Design review of the part built by this model. Coordinates are the model's own, in mm. Round coordinates to 2 decimals unless told otherwise and drop trailing zeros. Loops run counter-clockwise (first coordinate to the right, second up) from the corner with the lowest first, then second, coordinate; pieces in that order, holes last. Notation, with made-up numbers: M 83,-8 L 89,-8 A18 cw 89,19 Z; hole C 59.5,45 d1. An arc over 180 degrees is marked long. One line per item, written item: value. Start each with the question number.
Item 1: We need section C-C (y = 8). Write out the cut boundary in (x, z), then the cut area to 3 significant figures.
Item 2: We need section B-B (x = 0). Write out the cut boundary in (y, z), then the cut area to 3 significant figures.
Item 3: Clearance check with a flat-ended pin moving along its axis: pin 1 (2 mm diameter, centred on x = -4, y = -1, fed in from -Z). State where the tip first meets the part, or that it passes through.
Item 4: For line 1 along Y through (x, z) = (0.25, 1.25); line 2 along Y through (x, z) = (-8.75, 0.5); line 3 along Y through (x, z) = (-6, 0.9), list the stretches that pass through material, from the lowest coordinate up.
Item 5: We need section D-D (x = -8). Write out the cut boundary in (y, z).
Item 6: We need section A-A (y = 0). Write out the cut boundary in (x, z).
Autodesk Inventor part; units mm, degrees
ref_plane "YZ Plane" through (0, 0, 0) normal (1, 0, 0) x (0, 1, 0)
ref_plane "XZ Plane" through (0, 0, 0) normal (0, 1, 0) x (-1, 0, 0)
ref_plane "XY Plane" through (0, 0, 0) normal (0, 0, 1) x (1, 0, 0)
sketch "Sketch1" plane through (0, 0, 0) normal (0, 0, 1) x (1, 0, 0)
  circle A0 centre (0, 0) radius 40
  circle A1 centre (0, -8) radius 1.5
  circle A2 centre (8, 0) radius 1.5
  circle A3 centre (0, 8) radius 1.5
  circle A4 centre (-8, 0) radius 1.5
  circle A5 centre (0, -34) radius 1.5
  circle A6 centre (-3.0155, -32.086) radius 0.5
  circle A7 centre (2.9845, -36.086) radius 0.5
  line L0 (-15, -37.081) -> (-15, 37.081)
  line L1 (15, -37.081) -> (15, 37.081)
  dimension "d0" = 80
  dimension "d1" = 8
  dimension "d2" = 3
  dimension "d5" = 360
  dimension "d9" = 3
  dimension "d10" = 34
  dimension "d11" = 15
  dimension "d12" = 15
extrude "Extrusion1" add sketch "Sketch1" along normal blind 2 contours L1 A0 L0
properties part number "z roto base" material "Steel, Mild"
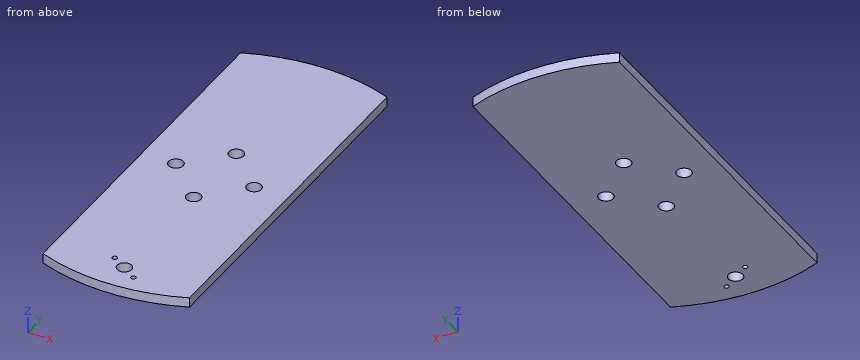
A:
1. outline: M -15,0 L -1.5,0 L -1.5,2 L -15,2 Z; M 1.5,0 L 15,0 L 15,2 L 1.5,2 Z
1. area: 54.0 mm2
2. outline: M -40,0 L -35.5,0 L -35.5,2 L -40,2 Z; M -32.5,0 L -9.5,0 L -9.5,2 L -32.5,2 Z; M -6.5,0 L 6.5,0 L 6.5,2 L -6.5,2 Z; M 9.5,0 L 40,0 L 40,2 L 9.5,2 Z
2. area: 142 mm2
3. pin 1: z = 0
4. line 1: -40 to -35.48, -32.52 to -9.48, -6.52 to 6.52, 9.48 to 40
4. line 2: -39.03 to -1.3, 1.3 to 39.03
4. line 3: -39.55 to 39.55
5. outline: M -39.19,0 L -1.5,0 L -1.5,2 L -39.19,2 Z; M 1.5,0 L 39.19,0 L 39.19,2 L 1.5,2 Z
6. outline: M -15,0 L -9.5,0 L -9.5,2 L -15,2 Z; M -6.5,0 L 6.5,0 L 6.5,2 L -6.5,2 Z; M 9.5,0 L 15,0 L 15,2 L 9.5,2 Z
